from build123d import *

# Parameters (mm, degrees)
F0_W     = 32.0802
F0_H     = 76.2
F1_DEPTH = 16.0401
F3_DEPTH = 32.0802


# Not quite as in the source:
# - a pattern or mirror of a feature is missing from the dataset's text; its kind, count and spacing are read off the source's solid


with BuildPart() as f1:
    # F0 (on Top) → F1 (new body, symmetric)
    with BuildSketch(Plane.XY):
        Rectangle(F0_W, F0_H)
    extrude(amount=F1_DEPTH, both=True)

    # F2 (on face) → F3 (cut, through all)
    with BuildSketch(Plane.XY.offset(16.0401)):
        Polygon((-16.0401, -38.1), (16.0401, -38.1), (16.0401, -6.0198), align=None)
    f3 = extrude(amount=-F3_DEPTH, mode=Mode.SUBTRACT)

    # F3_copies: F3 across plane
    add(f3.mirror(Plane.ZX), mode=Mode.SUBTRACT)


solid = f1.part
Part model, mm, in its own coordinate system. Give positions to 0.01 mm unless a question says otherwise; leave off trailing zeros. Loops run counter-clockwise (first coordinate to the right, second up) from the corner with the lowest first, then second, coordinate; pieces in that order, holes last.
(1) Drill centre lines: line 1 along X through (y, z) = (-14, -2.5); line 2 along Y through (x, z) = (8.5, -12); line 3 along Y through (x, z) = (13, -5.5). Where is each one in solid material? Low to high.
Return value:
line 1: x = -16.04 to 8.06
line 2: y = -13.56 to 13.56
line 3: y = -9.06 to 9.06
(2) Pin check, flat tips, straight feed: pin 1 (5 mm diameter, centred on x = 6.5, z = 12.5, fed in from +Y); pin 2 (1 mm diameter, centred on x = 3, z = 12.5, fed in from -Y); pin 3 (5 mm diameter, centred on x = 2.5, z = 11.5, fed in from +Y). Stop position of each tip, or through.
Return value:
pin 1: stops at y = 18.06
pin 2: stops at y = -19.56
pin 3: stops at y = 22.06
(3) Band-saw the part on B-B (x = -11). Write the cut outline in (y, z), and give its area (3 significant figures).
Return value:
outline: (-33.06, -16.04) - (33.06, -16.04) - (33.06, 16.04) - (-33.06, 16.04) - close
area: 2,120 mm2
(4) Band-saw the part on A-A (z = 4). Write the cut outline in (x, y), and give its area (3 significant figures).
Return value:
outline: (-16.04, -38.1) - (16.04, -6.02) - (16.04, 6.02) - (-16.04, 38.1) - close
area: 1,420 mm2
